Design review of the part built by this model. Coordinates are the model's own, in mm. Round coordinates to 2 decimals unless told otherwise and drop trailing zeros. Loops run counter-clockwise (first coordinate to the right, second up) from the corner with the lowest first, then second, coordinate; pieces in that order, holes last. Notation, with made-up numbers: (15.25, 27.25) - (74.25, 27.25) arc R10 cw to (74.25, 37.25) - close; hole circle Ø9 at (-28.75, -3). An arc over 180 degrees is marked (long way). Answer as CSV lines item,"result". Start each with the question number.
(1) Consider section B-B (y = 1.6). Count the separate pieces of the cut face and the enclosed holes in it, and give its area (3 significant figures).
(2) For P1, Ø1, axis at x = -37.5, y = 0.5, coming from the -Z side, flat-tipped, find the tip position at first contact; note if it passes through.
(3) Consider section A-A (z = 21.5). Give the boundary of the cut face in (x, y).
(4) Wall thickness on L1, parallel to X at y = 0.8, z = 90.5; L2, parallel to X at y = 2.1, z = 32; L3, parallel to X at y = 2.45, z = -0.5: over which ranges is each line inside the solid? List them lowest first.
from build123d import *

# Parameters (mm, degrees)
SKETCH_1_W              = 200
SKETCH_1_H              = 200
EXTRUDE_1_DEPTH         = 3
SKETCH_2_R              = 1.55
CUT_EXTRUDE_2_DEPTH     = 10
CUT_EXTRUDE_3_DEPTH     = 10
SKETCH_6_R              = 1.55
CUT_EXTRUDE_3_1_1_DEPTH = 10
SKETCH_9_R              = 4
CUT_EXTRUDE_5184_DEPTH  = 113.522220028
EXTRUDE_2_DEPTH         = 30
CUT_EXTRUDE_2006_REACH  = 141.862
SKETCH_10_R             = 4
CUT_EXTRUDE_6949_REACH  = 141.862
CUT_EXTRUDE_4_DEPTH     = 10
SKETCH_13_W             = 103
SKETCH_13_H             = 3
EXTRUDE_3_DEPTH         = 75
CUT_EXTRUDE_7474_DEPTH  = 10
HOLE_WIZARD_3_1_3_1_1_D = 3.1
FILLET_1_R              = 4
HOLE_WIZARD_3_1_3_1_2_D = 3.1


with BuildPart() as part:
    # 草图1 → 凸台-拉伸1 (new body)
    with BuildSketch(Plane(origin=(0, 0, 0), x_dir=(1, 0, 0), z_dir=(0, 1, 0))):
        Rectangle(SKETCH_1_W, SKETCH_1_H)
    extrude(amount=EXTRUDE_1_DEPTH)

    # 草图2 → 切除-拉伸2 (cut)
    with BuildSketch(Plane(origin=(0, 3, 0), x_dir=(1, 0, 0), z_dir=(0, 1, 0))):
        with Locations(Location((29.5, 9.5, 0), (0, 0, 270))):
            Circle(SKETCH_2_R)
        with Locations(Location((21.5, 0, 0), (0, 0, 270))):
            Circle(SKETCH_2_R)
        with Locations(Location((29.5, -9.5, 0), (0, 0, 270))):
            Circle(SKETCH_2_R)
        with Locations(Location((37.5, 0, 0), (0, 0, 270))):
            Circle(SKETCH_2_R)
        with Locations(Location((-29.5, -9.5, 0), (0, 0, 270))):
            Circle(SKETCH_2_R)
        with Locations(Location((-37.5, 0, 0), (0, 0, 270))):
            Circle(SKETCH_2_R)
        with Locations(Location((-21.5, 0, 0), (0, 0, 270))):
            Circle(SKETCH_2_R)
        with Locations(Location((-29.5, 9.5, 0), (0, 0, 270))):
            Circle(SKETCH_2_R)
        with Locations(Location((-15, -32, 0), (0, 0, 270))):
            Circle(SKETCH_2_R)
        with Locations(Location((15, -32, 0), (0, 0, 270))):
            Circle(SKETCH_2_R)
    extrude(amount=-CUT_EXTRUDE_2_DEPTH, mode=Mode.SUBTRACT)

    # 草图5 → 切除-拉伸3 (cut)
    with BuildSketch(Plane(origin=(0, 3, 0), x_dir=(1, 0, 0), z_dir=(0, 1, 0))):
        with BuildLine():
            Line((51.5, -0.0030003), (51.5, -100))
            Line((51.5, -100), (100, -100))
            Line((100, -100), (100, 100))
            Line((100, 100), (-100, 100))
            Line((-100, 100), (-100, -100))
            Line((-100, -100), (-51.5, -100))
            Line((-51.5, -100), (-51.5, -0.0030003))
            ThreePointArc((-51.5, -0.0030003), (-47.106601718, 10.603601418), (-36.5, 14.9969997))
            Line((-36.5, 14.9969997), (-29, 14.9969997))
            ThreePointArc((-29, 14.9969997), (-22.636038969, 17.633038669), (-20, 23.9969997))
            Line((-20, 23.9969997), (-20, 24.9949995))
            Line((-20, 24.9949995), (-20, 47.5))
            Line((-20, 47.5), (0, 47.5))
            Line((0, 47.5), (20, 47.5))
            Line((20, 47.5), (20, 24.9949995))
            Line((20, 24.9949995), (20, 23.9969997))
            ThreePointArc((20, 23.9969997), (22.636038969, 17.633038669), (29, 14.9969997))
            Line((29, 14.9969997), (36.5, 14.9969997))
            ThreePointArc((36.5, 14.9969997), (47.106601718, 10.603601418), (51.5, -0.0030003))
        make_face()
    extrude(amount=-CUT_EXTRUDE_3_DEPTH, mode=Mode.SUBTRACT)

    # 草图6 → φ3.1通孔1 (cut)
    with BuildSketch(Plane.XZ):
        with Locations(Location((-15, -42.5, 0), (0, 0, 270))):
            Circle(SKETCH_6_R)
        with Locations(Location((-15, -27.5, 0), (0, 0, 270))):
            Circle(SKETCH_6_R)
        with Locations(Location((15, -27.5, 0), (0, 0, 90))):
            Circle(SKETCH_6_R)
        with Locations(Location((15, -42.5, 0), (0, 0, 90))):
            Circle(SKETCH_6_R)
    extrude(amount=-CUT_EXTRUDE_3_1_1_DEPTH, mode=Mode.SUBTRACT)

    # 草图9 → Cut-Extrude 5184 (cut, through all)
    with BuildSketch(Plane(origin=(0, 3, 0), x_dir=(1, 0, 0), z_dir=(0, 1, 0))):
        with Locations(Location((0, -53.75, 0), (0, 0, 270))):
            Circle(SKETCH_9_R)
    extrude(amount=-CUT_EXTRUDE_5184_DEPTH, mode=Mode.SUBTRACT)

    # 草图11 → 凸台-拉伸2 (add)
    with BuildSketch(Plane.XY.offset(100)):
        Polygon((-44.5, 3), (-51.5, 3), (-51.5, 0), (-44.5, 0), (44.5, 0), (51.5, 0), (51.5, 3), (44.5, 3), align=None)
    extrude(amount=EXTRUDE_2_DEPTH)

    # 草图10 → 2006电机穿线孔 (cut, up to next)
    with BuildSketch(Plane.XZ, mode=Mode.PRIVATE) as cut_extrude_2006_sk1:
        with Locations(Location((-31.5, 21.5, 0), (0, 0, 270))):
            Circle(SKETCH_10_R)
    cut_extrude_2006_tool1 = extrude(cut_extrude_2006_sk1.sketch, amount=-CUT_EXTRUDE_2006_REACH, mode=Mode.PRIVATE) & part.part
    # 草图10 → 2006电机穿线孔 (cut, up to next)
    with BuildSketch(Plane.XZ, mode=Mode.PRIVATE) as cut_extrude_2006_sk2:
        with Locations(Location((31.5, 21.5, 0), (0, 0, 270))):
            Circle(SKETCH_10_R)
    cut_extrude_2006_tool2 = extrude(cut_extrude_2006_sk2.sketch, amount=-CUT_EXTRUDE_2006_REACH, mode=Mode.PRIVATE) & part.part
    add(cut_extrude_2006_tool1.solids().sort_by_distance((-31.5, 0, 21.5))[0], mode=Mode.SUBTRACT)
    add(cut_extrude_2006_tool2.solids().sort_by_distance((31.5, 0, 21.5))[0], mode=Mode.SUBTRACT)

    # 草图12 → Cut-Extrude 6949 (cut, up to next)
    with BuildSketch(Plane(origin=(0, 3, 0), x_dir=(1, 0, 0), z_dir=(0, 1, 0)), mode=Mode.PRIVATE) as cut_extrude_6949_sk1:
        with BuildLine():
            Line((-9.7, -64.7), (9.7, -64.7))
            ThreePointArc((9.7, -64.7), (10.407106781, -64.992893219), (10.7, -65.7))
            Line((10.7, -65.7), (10.7, -70.08))
            ThreePointArc((10.7, -70.08), (10.407106781, -70.787106781), (9.7, -71.08))
            Line((9.7, -71.08), (-9.7, -71.08))
            ThreePointArc((-9.7, -71.08), (-10.407106781, -70.787106781), (-10.7, -70.08))
            Line((-10.7, -70.08), (-10.7, -65.7))
            ThreePointArc((-10.7, -65.7), (-10.407106781, -64.992893219), (-9.7, -64.7))
        make_face()
    cut_extrude_6949_tool1 = extrude(cut_extrude_6949_sk1.sketch, amount=-CUT_EXTRUDE_6949_REACH, mode=Mode.PRIVATE) & part.part
    add(cut_extrude_6949_tool1.solids().sort_by_distance((0, 3, 67.89))[0], mode=Mode.SUBTRACT)

    # 草图7 → 切除-拉伸4 (cut)
    with BuildSketch(Plane(origin=(0, 3, 0), x_dir=(1, 0, 0), z_dir=(0, 1, 0))):
        with BuildLine():
            Line((-49.05, -70), (-49.05, -60))
            ThreePointArc((-49.05, -60), (-47.5, -58.45), (-45.95, -60))
            Line((-45.95, -60), (-45.95, -70))
            ThreePointArc((-45.95, -70), (-47.5, -71.55), (-49.05, -70))
        make_face()
        with BuildLine():
            Line((-49.05, -92), (-49.05, -82))
            ThreePointArc((-49.05, -82), (-47.5, -80.45), (-45.95, -82))
            Line((-45.95, -82), (-45.95, -92))
            ThreePointArc((-45.95, -92), (-47.5, -93.55), (-49.05, -92))
        make_face()
        with BuildLine():
            Line((45.95, -92), (45.95, -82))
            ThreePointArc((45.95, -82), (47.5, -80.45), (49.05, -82))
            Line((49.05, -82), (49.05, -92))
            ThreePointArc((49.05, -92), (47.5, -93.55), (45.95, -92))
        make_face()
        with BuildLine():
            Line((45.95, -70), (45.95, -60))
            ThreePointArc((45.95, -60), (47.5, -58.45), (49.05, -60))
            Line((49.05, -60), (49.05, -70))
            ThreePointArc((49.05, -70), (47.5, -71.55), (45.95, -70))
        make_face()
    extrude(amount=-CUT_EXTRUDE_4_DEPTH, mode=Mode.SUBTRACT)

    # 草图13 → 凸台-拉伸3 (add)
    with BuildSketch(Plane.XY.offset(130)):
        with Locations((0, 1.5)):
            Rectangle(SKETCH_13_W, SKETCH_13_H)
    extrude(amount=EXTRUDE_3_DEPTH)

    # 草图14 → Cut-Extrude 7474 (cut)
    with BuildSketch(Plane(origin=(0, 3, 0), x_dir=(1, 0, 0), z_dir=(0, 1, 0))):
        with BuildLine():
            Line((-15, -90.75), (15, -90.75))
            ThreePointArc((15, -90.75), (18, -93.75), (15, -96.75))
            Line((15, -96.75), (-15, -96.75))
            ThreePointArc((-15, -96.75), (-18, -93.75), (-15, -90.75))
        make_face()
    extrude(amount=-CUT_EXTRUDE_7474_DEPTH, mode=Mode.SUBTRACT)

    # Ø3.1 (3.1) 直径孔1 (through all)
    with Locations(Plane(origin=(-47.5, 3, 120), x_dir=(0, 0, 1), z_dir=(0, 1, 0))):
        with Locations((0, 0), (0, 95), (55, 0), (55, 95)):
            Hole(HOLE_WIZARD_3_1_3_1_1_D / 2)

    # 圆角1
    fillet_1_edges = [part.edges().sort_by_distance(p)[0] for p in [
        (-51.5, 1.5, 205),
        (51.5, 1.5, 205),
    ]]
    fillet(fillet_1_edges, radius=FILLET_1_R)

    # Ø3.1 (3.1) 直径孔2 (through all)
    with Locations(Plane(origin=(-15, 3, 102), x_dir=(0, 0, 1), z_dir=(0, 1, 0))):
        with Locations((0, 0), (0, 30), (70, 0)):
            Hole(HOLE_WIZARD_3_1_3_1_2_D / 2)


solid = part.part
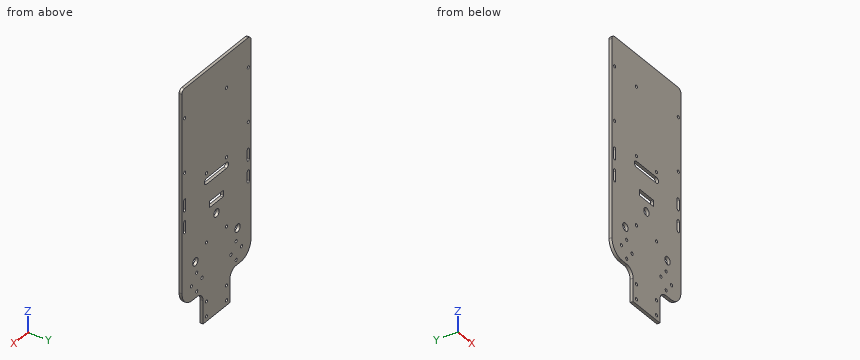
Determined:
1,separate pieces,"1"
1,enclosed holes,"30"
1,area,"23,100 mm^2"
2,P1,"stops at z = -14.99"
3,outline,"(-51.5, 0) - (-35.5, 0) - (-35.5, 3) - (-51.5, 3) - close; (-27.5, 0) - (27.5, 0) - (27.5, 3) - (-27.5, 3) - close; (35.5, 0) - (51.5, 0) - (51.5, 3) - (35.5, 3) - close"
4,L1,"x = -51.5 to -49.05, -45.95 to 45.95, 49.05 to 51.5"
4,L2,"x = -51.5 to -16.55, -13.45 to 13.45, 16.55 to 51.5"
4,L3,"x = -51.49 to -38.97, -36.03 to -22.97, -20.03 to 20.03, 22.97 to 36.03, 38.97 to 51.49"
